Answer from the drawing. Dimensions are ordinates in mm from the lowest x, y and z of the part. A direction names the side the tool comes from. Coordinates: 2 decimals unless noted, no trailing zeros. Write each loop counter-clockwise with the first axis right and the second up, starting at its lowest first coordinate (ties: lowest second). Pieces come first, ordered by that corner, then holes.
1) The part is cut by section C-C (x = 48). Determine the outline of the cut face in (y, z).
2) The part is cut by section B-B (z = 6.5). Determine the outline of the cut face in (x, y).
3) Each of these flat-tipped pins is pushed along its axis until it touches: pin 1 Ø1.5 at (y, z) = (32, 36) entering from -X; pin 2 Ø5 at (x, y) = (21.5, 4) entering from +Z; pin 3 Ø18.5 at (x, y) = (20, 31.5) entering from +Z. Where does it stop, or does it pass through?
4) The part is cut by section A-A (y = 6.5). Determine the outline of the cut face in (x, z), then the cut area to 3 significant figures.
5) Find the intervals of material crossed by line 1 (X direction, y = 37.5, z = 34.5); line 2 (X direction, y = 8, z = 8.5); line 3 (Z direction, x = 33, y = 32), in increasing order.
6) The part is cut by section D-D (y = 40). Determine the outline of the cut face in (x, z), then the cut area to 3 significant figures.
7) Which of the six approach directions +Z, -Z, +X, -X, +Y, -Y give full straight-line access (tool end or side, diameter ignored) to the marked faces 1, 2 and 3?
8) Determine the mould class of the marked faces 4, 5, 6 and 7 for opening direction X: +X half, -X half, draft (parallel to the pull), parting line (faces both ways), or undercut.
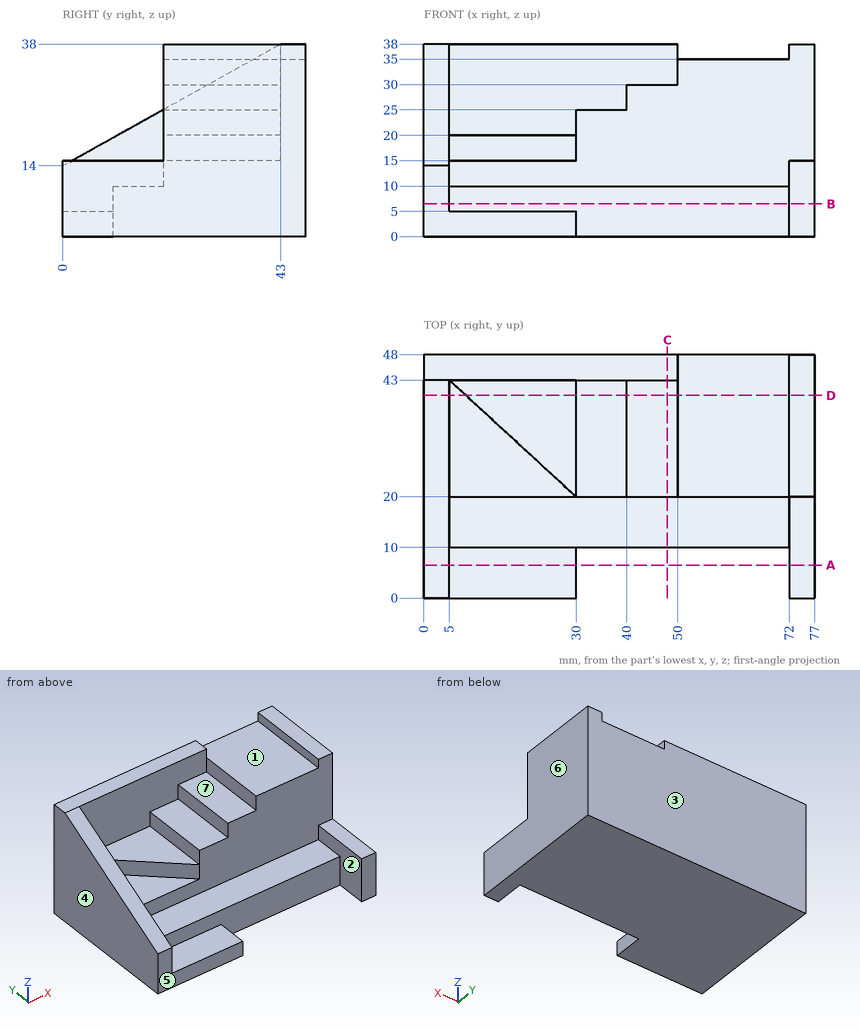
Reported:
1. outline: (10, 0) - (48, 0) - (48, 38) - (43, 38) - (43, 30) - (20, 30) - (20, 10) - (10, 10) - close
2. outline: (0, 0) - (5, 0) - (5, 10) - (72, 10) - (72, 0) - (77, 0) - (77, 48) - (0, 48) - close
3. pin 1: stops at x = 72
3. pin 2: stops at z = 5
3. pin 3: stops at z = 20
4. outline: (0, 0) - (30, 0) - (30, 5) - (5, 5) - (5, 17.63) - (0, 17.63) - close; (72, 0) - (77, 0) - (77, 15) - (72, 15) - close
4. area: 288 mm2
5. line 1: x = 0 to 5, 50 to 77
5. line 2: x = 0 to 5, 72 to 77
5. line 3: z = 0 to 25
6. outline: (0, 0) - (77, 0) - (77, 38) - (72, 38) - (72, 35) - (50, 35) - (50, 30) - (40, 30) - (40, 25) - (30, 25) - (30, 20) - (8.26, 20) - (8.26, 15) - (5, 15) - (5, 36.33) - (0, 36.33) - close
6. area: 2,180 mm2
7. face 1: +Z, +Y, -Y
7. face 2: +Z, -Y
7. face 3: +Z, -Z, +X, -X, +Y
8. face 4: -X half
8. face 5: draft
8. face 6: +X half
8. face 7: undercut
